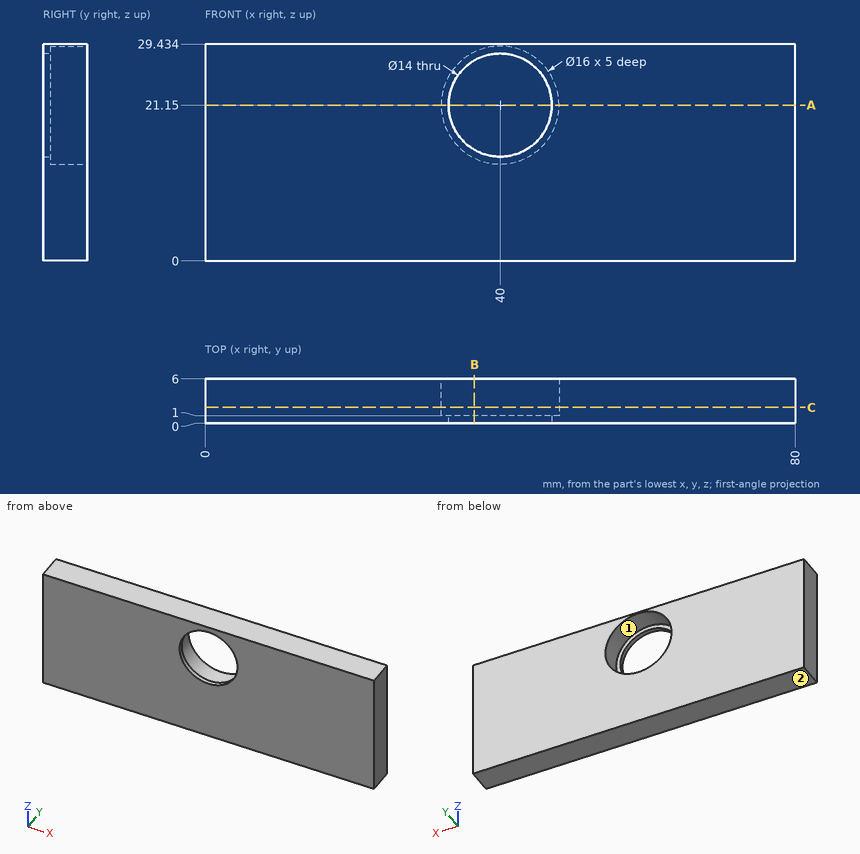
For this review, use the dimensioned drawing (mm, ordinates from the lowest corner) and the shaded views. Coordinates: 2 decimals unless noted, no trailing zeros. Order: outer loops, then holes, each group sorted by start corner. A loop starts at its lowest first (then second) coordinate and runs counter-clockwise, first axis right, second up. Notation, with made-up numbers: M 28,82 L 35,82 A26 ccw 35,105 Z; hole C 53.5,-19 d9. An arc over 180 degrees is marked long. Answer as a JSON object with one key per item and string values. Group by question number.
1) Wall thickness on L1, parallel to X at y = 0.6, z = 21.15; L2, parallel to Z at x = 40, y = 2.9; L3, parallel to X at y = 0.75, z = 20: over which ranges is each line inside the solid? List them lowest first.
2) Add section A-A, the plane z = 21.15. Write out the cut boundary in (x, y).
3) Add section C-C, the plane y = 2.15. Write out the cut boundary in (x, z).
4) Mouldability with a two-part tool opening along X and no side actions: class the marked faces 1 and 2 as pulls with the +X half, pulls with the -X half, needs draft (parallel to the pull), parting line crosses it, or undercut.
5) Add section B-B, the plane x = 36.5. Write out the cut boundary in (y, z), then the cut area to 3 significant figures.
6) For pin 1 (9.5 mm diameter, centred on x = 40, z = 21.15, fed in from -Y), flat-tipped, find the tip position at first contact; note if it passes through.
Computed values:
{
 "1": {"L1": "x = 0 to 33, 47 to 80", "L2": "z = 0 to 13.15, 29.15 to 29.43", "L3": "x = 0 to 33.1, 46.9 to 80"},
 "2": {"outline": "M 0,0 L 33,0 L 33,1 L 32,1 L 32,6 L 0,6 Z; M 47,0 L 80,0 L 80,6 L 48,6 L 48,1 L 47,1 Z"},
 "3": {"outline": "M 0,0 L 80,0 L 80,29.43 L 0,29.43 Z; hole C 40,21.15 d16"},
 "4": {"face 1": "undercut", "face 2": "needs draft"},
 "5": {"outline": "M 0,0 L 6,0 L 6,13.96 L 1,13.96 L 1,15.09 L 0,15.09 Z; M 0,27.21 L 1,27.21 L 1,28.34 L 6,28.34 L 6,29.43 L 0,29.43 Z", "area": "92.5 mm^2"},
 "6": {"pin 1": "passes through"}
}
